from build123d import *

# Parameters (mm, degrees)
EXTRU_MINCE1_DEPTH      = 35
CONG_1_R                = 2
CONG_3_R                = 1
ESQUISSE3_R             = 1.75
ESQUISSE3_R_2           = 3.5
ENL_V_MAT_EXTRU_2_DEPTH = 2
CONG_5_R                = 2
CONG_6_R                = 2
CONG_7_R                = 2
CONG_8_R                = 2
ESQUISSE4_R             = 1.75
ENL_V_MAT_EXTRU_3_DEPTH = 2


with BuildPart() as part:
    # Esquisse1 → Extru.-Mince1 (new body)
    with BuildSketch(Plane.XY):
        Polygon((0, 0), (58, 0), (58, 65), (60, 65), (60, -2), (0, -2), align=None)
    extrude(amount=EXTRU_MINCE1_DEPTH)

    # Congé1
    cong_1_edges = [part.edges().sort_by_distance(p)[0] for p in [
        (60, -2, 17.5),
    ]]
    fillet(cong_1_edges, radius=CONG_1_R)

    # Congé3
    cong_3_edges = [part.edges().sort_by_distance(p)[0] for p in [
        (58, 0, 17.5),
    ]]
    fillet(cong_3_edges, radius=CONG_3_R)

    # Esquisse3 → Enlèv. mat.-Extru.2 (cut)
    with BuildSketch(Plane(origin=(60, 0, 0), x_dir=(0, 0, -1), z_dir=(1, 0, 0))):
        with Locations((-17.5, 35.5)):
            Circle(ESQUISSE3_R)
        with Locations((-17.5, 54.5)):
            Circle(ESQUISSE3_R)
        with Locations((-17.5, 45)):
            Circle(ESQUISSE3_R_2)
    extrude(amount=-ENL_V_MAT_EXTRU_2_DEPTH, mode=Mode.SUBTRACT)

    # Congé5
    cong_5_edges = [part.edges().sort_by_distance(p)[0] for p in [
        (59, 65, 35),
    ]]
    fillet(cong_5_edges, radius=CONG_5_R)

    # Congé6
    cong_6_edges = [part.edges().sort_by_distance(p)[0] for p in [
        (59, 65, 0),
    ]]
    fillet(cong_6_edges, radius=CONG_6_R)

    # Congé7
    cong_7_edges = [part.edges().sort_by_distance(p)[0] for p in [
        (0, -1, 0),
    ]]
    fillet(cong_7_edges, radius=CONG_7_R)

    # Congé8
    cong_8_edges = [part.edges().sort_by_distance(p)[0] for p in [
        (0, -1, 35),
    ]]
    fillet(cong_8_edges, radius=CONG_8_R)

    # Esquisse4 → Enlèv. mat.-Extru.3 (cut)
    with BuildSketch(Plane(origin=(0, 0, 0), x_dir=(1, 0, 0), z_dir=(0, 1, 0))):
        with Locations(Location((26, -17.5, 0), (0, 0, 270))):
            Circle(ESQUISSE4_R)
        with Locations(Location((14, -17.5, 0), (0, 0, 270))):
            Circle(ESQUISSE4_R)
    extrude(amount=-ENL_V_MAT_EXTRU_3_DEPTH, mode=Mode.SUBTRACT)


solid = part.part
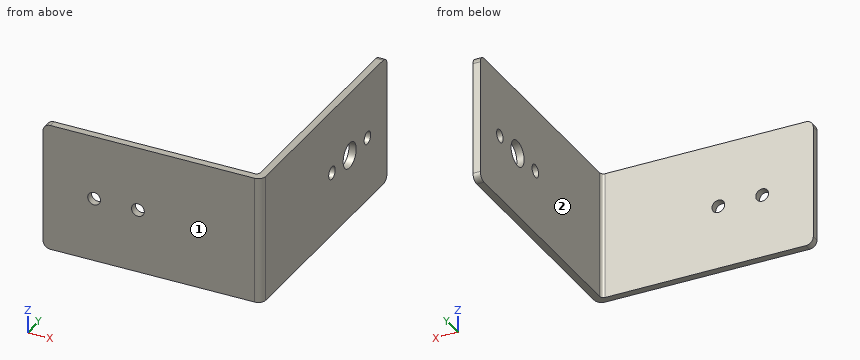
Can you work these out from the model? Positions are in its coordinate system, mm. Face numbers are marked on the shaded views. A direction names the side the tool comes from. Coordinates: 2 decimals unless noted, no trailing zeros. Write each loop counter-clockwise with the first axis right and the second up, starting at its lowest first coordinate (ties: lowest second). Pieces come first, ordered by that corner, then holes.
Q1. Imagine slicing it at A-A, the plane x = 14. List the corners of the cut face in (y, z) for me, plus the area to 3 significant figures.
Results found:
outline: (-2, 0) - (0, 0) - (0, 15.75) - (-2, 15.75) - close; (-2, 19.25) - (0, 19.25) - (0, 35) - (-2, 35) - close
area: 63.0 mm2
Q2. Which directions (+Z, -Z, +X, -X, +Y, -Y) give clear straight access to the entire face, cutting with the end or side of a thin tool? Please do the marked faces 1 and 2.
Results found:
face 1: +Z, -Z, +X, -X, -Y
face 2: +Z, -Z, -X, +Y
Q3. Imagine slicing it at B-B, the plane y = 45. List the corners of the cut face in (x, z) for me, plus the area to 3 significant figures.
Results found:
outline: (58, 0) - (60, 0) - (60, 14) - (58, 14) - close; (58, 21) - (60, 21) - (60, 35) - (58, 35) - close
area: 56.0 mm2
Q4. Please list where these lines run through material, in increasing order: L1, parallel to X at y = -1.4, z = 17.5; L2, parallel to Y at x = 59, z = 17; L3, parallel to Y at x = 36.5, z = 2.
Results found:
L1: x = 0 to 12.25, 15.75 to 24.25, 27.75 to 59.43
L2: y = -1.73 to 33.82, 37.18 to 41.54, 48.46 to 52.82, 56.18 to 65
L3: y = -2 to 0
Q5. Imagine slicing it at C-C, the plane z = 17.5. List the corners of the cut face in (x, y) for me.
Results found:
outline: (0, -2) - (12.25, -2) - (12.25, 0) - (0, 0) - close; (15.75, -2) - (24.25, -2) - (24.25, 0) - (15.75, 0) - close; (27.75, -2) - (58, -2) arc R2 ccw to (60, 0) - (60, 33.75) - (58, 33.75) - (58, 1) arc R1 cw to (57, 0) - (27.75, 0) - close; (58, 37.25) - (60, 37.25) - (60, 41.5) - (58, 41.5) - close; (58, 48.5) - (60, 48.5) - (60, 52.75) - (58, 52.75) - close; (58, 56.25) - (60, 56.25) - (60, 65) - (58, 65) - close
Q6. For P1, Ø10.5, axis at y = 25, z = 20, coming from the -X side; P2, Ø4.5, axis at x = 14, z = 17.5, coming from the +Y side, each with a flat end and sliding along its axis, tell me the tip position at first contact or that it passes through.
Results found:
P1: stops at x = 58
P2: stops at y = 0
Q7. Imagine slicing it at D-D, the plane z = 12. List the corners of the cut face in (x, y) for me.
Results found:
outline: (0, -2) - (58, -2) arc R2 ccw to (60, 0) - (60, 65) - (58, 65) - (58, 1) arc R1 cw to (57, 0) - (0, 0) - close
